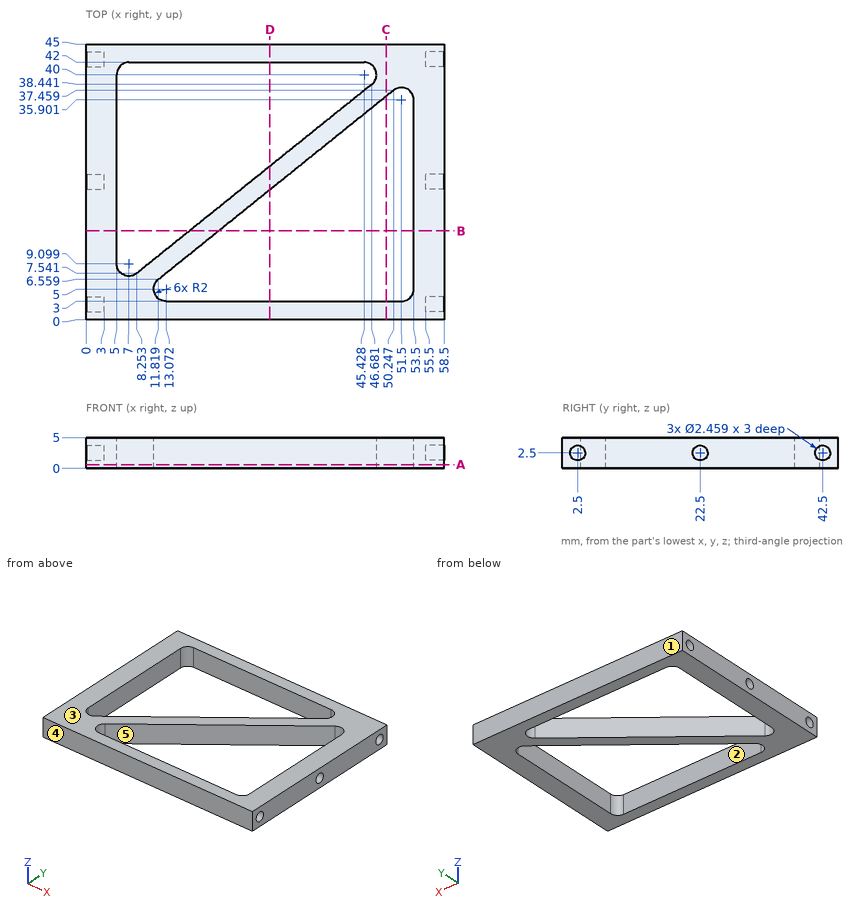
Job drawing, mm, ordinate dimensions from the low corner. One solid piece. A direction names the side the tool comes from. Coordinates: 2 decimals unless noted, no trailing zeros. Order: outer loops, then holes, each group sorted by start corner. A loop starts at its lowest first (then second) coordinate and runs counter-clockwise, first axis right, second up. Notation, with made-up numbers: (5.25, -38.75) -> (17.25, -38.75) arc R24 cw to (17.25, -14.75) -> close; hole circle Ø9 at (-10.5, 43.5). An arc over 180 degrees is marked (long way). Answer in a Markdown table with one row per item. Add a question column.
Q1. Wall check: line 1 along Y through (x, z) = (1.25, 2.5); line 2 along Z through (x, y) = (0.7, 2.5); line 3 along Y through (x, z) = (7, 3.25). Give the ranges that are in metal, low to high. Write a range as [from, to].
Q2. Band-saw the part on D-D, the plane x = 30. List the corners of the cut face in (y, z).
Q3. Mould opens along Y. For the marked faces 1, 2 and 3 say: +Y half, -Y half, draft (parallel to the pull), parting line (faces both ways), or undercut.
Q4. Band-saw the part on B-B, the plane y = 14.5. List the corners of the cut face in (x, z) (1 decimal).
Q5. Band-saw the part on C-C, the plane x = 49. List the corners of the cut face in (y, z).
Q6. Band-saw the part on A-A, the plane z = 0.6. List the corners of the cut face in (x, y).
Q7. Drop flat-ended pins along their axis: pin 1 (2.5 mm diameter, centred on x = 29, z = 2, fed in from -Y); pin 2 (1.5 mm diameter, centred on y = 2.5, z = 2.5, fed in from +X); pin 3 (1.5 mm diameter, centred on y = 42.5, z = 2.5, fed in from -X); pin 4 (10 mm diameter, centred on x = 40.5, y = 11, fed in from +Z). Give the stop position or say it passes through.
Q8. Which spindle directions (+Z, -Z, +X, -X, +Y, -Y) get a long thin tool onto all of the face, cutting with end or side? Do the marked faces 4 and 5. Say none if no direction does.
Answers follow:
| question | item | result |
|---|---|---|
| 1 | line 1 | [0, 1.27], [3.73, 21.27], [23.73, 41.27], [43.73, 45] |
| 1 | line 2 | [0, 1.27], [3.73, 5] |
| 1 | line 3 | [0, 7.1], [42, 45] |
| 2 | outline | (0, 0) -> (3, 0) -> (3, 5) -> (0, 5) -> close; (21.18, 0) -> (25.03, 0) -> (25.03, 5) -> (21.18, 5) -> close; (42, 0) -> (45, 0) -> (45, 5) -> (42, 5) -> close |
| 3 | face 1 | +Y half |
| 3 | face 2 | undercut |
| 3 | face 3 | draft |
| 4 | outline | (0, 0) -> (5, 0) -> (5, 5) -> (0, 5) -> close; (16.9, 0) -> (21.7, 0) -> (21.7, 5) -> (16.9, 5) -> close; (53.5, 0) -> (58.5, 0) -> (58.5, 5) -> (53.5, 5) -> close |
| 5 | outline | (0, 0) -> (3, 0) -> (3, 5) -> (0, 5) -> close; (36.46, 0) -> (45, 0) -> (45, 5) -> (36.46, 5) -> close |
| 6 | outline | (0, 0) -> (58.5, 0) -> (58.5, 45) -> (0, 45) -> close; hole (5, 9.1) arc R2 ccw to (8.25, 7.54) -> (46.68, 38.44) arc R2 ccw to (45.43, 42) -> (7, 42) arc R2 ccw to (5, 40) -> close; hole (11.82, 6.56) arc R2 ccw to (13.07, 3) -> (51.5, 3) arc R2 ccw to (53.5, 5) -> (53.5, 35.9) arc R2 ccw to (50.25, 37.46) -> close |
| 7 | pin 1 | y = 0 |
| 7 | pin 2 | x = 55.5 |
| 7 | pin 3 | x = 3 |
| 7 | pin 4 | through |
| 8 | face 4 | +Z, -Z, +X, -X, -Y |
| 8 | face 5 | +Z, -Z |
